Part model, mm, in its own coordinate system. Give positions to 0.01 mm unless a question says otherwise; leave off trailing zeros. Loops run counter-clockwise (first coordinate to the right, second up) from the corner with the lowest first, then second, coordinate; pieces in that order, holes last. Notation, with made-up numbers: (36, 28) -> (60, 28) arc R23 cw to (60, 66) -> close; hole circle Ø4 at (5.25, 87). An arc over 180 degrees is marked (long way). One line per question, with ' | ' between items.
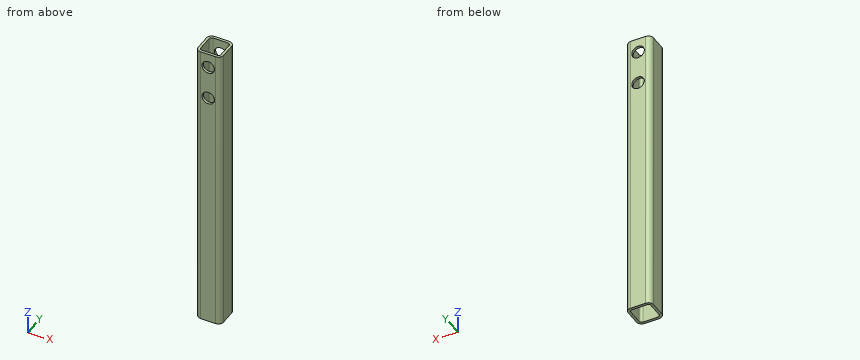
Autodesk Inventor part; units mm, degrees
ref_plane "Piano iniziale" through (0, 0, 0) normal (0, 0, 1) x (1, 0, 0)
ref_plane "Piano finale" through (0, 0, 235) normal (0, 0, 1) x (1, 0, 0)
ref_plane "YZ Plane" through (0, 0, 0) normal (1, 0, 0) x (0, 1, 0)
ref_plane "Piano iniziale" through (0, 0, 0) normal (0, 0, 1) x (1, 0, 0)
ref_plane "Piano finale" through (0, 0, 235) normal (0, 0, 1) x (1, 0, 0)
sketch "Schizzo" plane through (0, 0, 0) normal (0, 0, 1) x (1, 0, 0)
  line L0 (-10, -6) -> (-10, 6)
  line L1 (-6, 10) -> (6, 10)
  line L2 (10, 6) -> (10, -6)
  line L3 (6, -10) -> (-6, -10)
  arc A0 (-10, -6) -> (-6, -10) centre (-6, -6) ccw
  arc A1 (10, 6) -> (6, 10) centre (6, 6) ccw
  arc A2 (-6, 10) -> (-10, 6) centre (-6, 6) ccw
  arc A3 (6, -10) -> (10, -6) centre (6, -6) ccw
  arc A4 (-6, 8) -> (-8, 6) centre (-6, 6) ccw
  line L4 (-6, 8) -> (6, 8)
  arc A5 (8, 6) -> (6, 8) centre (6, 6) ccw
  line L5 (8, 6) -> (8, -6)
  arc A6 (6, -8) -> (8, -6) centre (6, -6) ccw
  line L6 (6, -8) -> (-6, -8)
  arc A7 (-8, -6) -> (-6, -8) centre (-6, -6) ccw
  line L7 (-8, -6) -> (-8, 6)
  line L8 (0, 15.1598) -> (0, -15.1598) construction
  line L9 (-15.1598, 0) -> (15.1598, 0) construction
  dimension "d7" = 4
  dimension "d9" = 20
  dimension "d11" = 20
  dimension "d12" = 2
  dimension "d15" = 10
  dimension "d16" = 10
extrude "Corpo" add sketch "Schizzo" along normal up to surface (235 mm away) from surface at 0
sketch "Sketch3" plane through (0, 0, 0) normal (0, 0, 1) x (1, 0, 0)
  line L0 (0, 0) -> (10, 0)
ref_plane "Work Plane3" through (0, 0, 0) normal (0, -1, 0) x (1, 0, 0)
sketch "Sketch4" plane through (0, 0, 0) normal (0, -1, 0) x (1, 0, 0)
  line L0 (-2, 0) -> (12, 0)
  line L1 (-2, 235) -> (12, 235)
  dimension "d18" = 235
sketch "Schizzo5" plane through (6, 10, 235) normal (0, 1, 0) x (1, 0, 0)
  line L0 (-12, 0) -> (0, 0)
  line L1 (4, 235) -> (4, 0)
  point P0 (-6, 235)
  point P1 (-5.9124, 11.5)
  point P2 (-5.9124, 38.5)
  dimension "d26" = 11.5
  dimension "d27" = 27
  dimension "d28" = 9.9124
hole "Foro1" at (0.0876, 10, 223.5) at (0.0876, 10, 196.5) direction (0, -1, 0) diameter 10 end through all
equation "\"d7\" = G_IR"
equation "\"d9\" = G_W"
equation "\"d11\" = G_H"
equation "\"d12\" = G_T"
equation "\"d15\" = 0.5 * d9"
equation "\"d16\" = 0.5 * d11"
equation "\"d3\" = G_L"
equation "\"G_W\" = 20"
equation "\"G_H\" = 20"
equation "\"G_T\" = 2"
equation "\"G_IR\" = 4"
equation "\"G_L\" = d18"
equation "\"G_OFFSET_START\" = 0"
equation "\"G_OFFSET_END\" = 0"
equation "\"d14\" = G_OFFSET_END + B_L"
equation "\"B_L\" = 235"
properties part number "ISO 10799-2 - 20x20x2 - 235" material "Acciaio, Dolce"
1) Saw through at C-C (z = 196.5). Give the cut face in (x, y), and give its area (3 significant figures).
Found:
outline: (-10, -6) arc R4 ccw to (-6, -10) -> (-4.91, -10) -> (-4.91, -8) -> (-6, -8) arc R2 cw to (-8, -6) -> (-8, 6) arc R2 cw to (-6, 8) -> (-4.91, 8) -> (-4.91, 10) -> (-6, 10) arc R4 ccw to (-10, 6) -> close; (5.09, -10) -> (6, -10) arc R4 ccw to (10, -6) -> (10, 6) arc R4 ccw to (6, 10) -> (5.09, 10) -> (5.09, 8) -> (6, 8) arc R2 cw to (8, 6) -> (8, -6) arc R2 cw to (6, -8) -> (5.09, -8) -> close | area: 93.7 mm2
2) Saw through at A-A (z = 53.5). Give the cut face in (x, y), and give its area (3 significant figures).
Found:
outline: (-10, -6) arc R4 ccw to (-6, -10) -> (6, -10) arc R4 ccw to (10, -6) -> (10, 6) arc R4 ccw to (6, 10) -> (-6, 10) arc R4 ccw to (-10, 6) -> close; hole (-8, -6) arc R2 ccw to (-6, -8) -> (6, -8) arc R2 ccw to (8, -6) -> (8, 6) arc R2 ccw to (6, 8) -> (-6, 8) arc R2 ccw to (-8, 6) -> close | area: 134 mm2
3) Drill centre lines: line 1 (Y direction, x = -4, z = 105); line 2 (X direction, y = -8.9, z = 196.5) (3 decimals). Where is each one in solid material? Low to high.
Found:
line 1: -10 to -8, 8 to 10 | line 2: -8.755 to -4.912, 5.088 to 8.755
4) Saw through at B-B (y = -3.75). Give the cut face in (x, z), and give its area (3 significant figures).
Found:
outline: (-10, 0) -> (-8, 0) -> (-8, 235) -> (-10, 235) -> close; (8, 0) -> (10, 0) -> (10, 235) -> (8, 235) -> close | area: 940 mm2
5) Pin check, flat tip, straight feed: P1, Ø2, axis at y = -7.5, z = 38, coming from the +X side. Stop position of the tip, or through.
Found:
P1: x = 9.97
6) Saw through at D-D (x = 2). Give the cut face in (y, z), and give its area (3 significant figures).
Found:
outline: (-10, 0) -> (-8, 0) -> (-8, 191.88) -> (-10, 191.88) -> close; (-10, 201.12) -> (-8, 201.12) -> (-8, 218.88) -> (-10, 218.88) -> close; (-10, 228.12) -> (-8, 228.12) -> (-8, 235) -> (-10, 235) -> close; (8, 0) -> (10, 0) -> (10, 191.88) -> (8, 191.88) -> close; (8, 201.12) -> (10, 201.12) -> (10, 218.88) -> (8, 218.88) -> close; (8, 228.12) -> (10, 228.12) -> (10, 235) -> (8, 235) -> close | area: 866 mm2
